Work out the finished part from the listing and answer in its coordinate system (mm). Give positions to 0.01 mm unless a question says otherwise; leave off trailing zeros. Loops run counter-clockwise (first coordinate to the right, second up) from the corner with the lowest first, then second, coordinate; pieces in that order, holes last. Notation, with made-up numbers: M -29,81.5 L -7,81.5 A23 cw -7,113.5 Z; hole C 45.5,0 d6. An arc over 180 degrees is marked long. Answer as a JSON object with one key per item and string values. Group by question number.
```python
from build123d import *

# Parameters (mm, degrees)
SKETCH1_W           = 25
SKETCH1_H           = 95
BOSS_EXTRUDE1_DEPTH = 1
BOSS_EXTRUDE2_START = -0.5
SKETCH3_W           = 3
SKETCH3_H           = 1
SKETCH3_W_2         = 1
SKETCH3_H_2         = 3
BOSS_EXTRUDE2_DEPTH = 0.5
SKETCH4_R           = 5
CUT_EXTRUDE1_DEPTH  = 1


with BuildPart() as part:
    # Sketch1 → Boss-Extrude1 (new body)
    with BuildSketch(Plane.XZ.offset(-34.2740501)):
        with Locations((-81.601257217, 49.307503177)):
            Rectangle(SKETCH1_W, SKETCH1_H)
    extrude(amount=-BOSS_EXTRUDE1_DEPTH)

    # Sketch3 → Boss-Extrude2 (add)
    with BuildSketch(Plane.XZ.offset(-34.2740501).offset(BOSS_EXTRUDE2_START)):
        with Locations((-81.601257217, 96.807503177)):
            Rectangle(SKETCH3_W, SKETCH3_H)
        with Locations((-94.101257217, 68.580262086)):
            Rectangle(SKETCH3_W_2, SKETCH3_H_2)
        with Locations((-94.101257217, 43.580262086)):
            Rectangle(SKETCH3_W_2, SKETCH3_H_2)
        with Locations((-94.101257217, 18.580262086)):
            Rectangle(SKETCH3_W_2, SKETCH3_H_2)
        with Locations((-69.101257217, 18.580262086)):
            Rectangle(SKETCH3_W_2, SKETCH3_H_2)
        with Locations((-69.101257217, 43.580262086)):
            Rectangle(SKETCH3_W_2, SKETCH3_H_2)
        with Locations((-69.101257217, 68.580262086)):
            Rectangle(SKETCH3_W_2, SKETCH3_H_2)
    extrude(amount=-BOSS_EXTRUDE2_DEPTH)

    # Sketch4 → Cut-Extrude1 (cut)
    with BuildSketch(Plane.XZ.offset(-34.2740501)):
        with Locations((-81.601257217, 1.807503177)):
            Circle(SKETCH4_R)
    extrude(amount=-CUT_EXTRUDE1_DEPTH, mode=Mode.SUBTRACT)


solid = part.part
```
Item 1: For a pull along X with two mould halves and no side action, classify faces 1 (the cylindrical face through (-81.491, 34.767, 6.806)), 2 (the flat face through (-82, 35.274, 50)) as pulls with the +X half, pulls with the -X half, needs draft (parallel to the pull), parting line crosses it, or undercut.
Item 2: Find the intervals of material crossed by probe 1 along Z at (x, y) = (-74.75, 35.2); probe 2 along X at (y, z) = (34.9, 38.5); probe 3 along X at (y, z) = (34.65, 6), in increasing order. Write a range as [from, to].
Item 3: Given pin 1 Ø0.6 at (x, y) = (-94.5, 35) entering from -Z; pin 2 Ø0.5 at (x, y) = (-76, 34.5) entering from +Z, each flat-ended and moving along its own axis, determine where each tip first touches the part or whether it passes through.
Item 4: A cutting plane is placed at C-C (x = -81.5). Determine the outline of the cut face in (y, z), and give its area (3 significant figures).
Item 5: A cutting plane is placed at D-D (x = -85.75). Determine the outline of the cut face in (y, z), and give its area (3 significant figures).
Item 6: A cutting plane is placed at B-B (z = 64.5). Determine the outline of the cut face in (x, y), and give its area (3 significant figures).
The answers:
{
 "1": {"face 1": "undercut", "face 2": "needs draft"},
 "2": {"probe 1": "z = [1.81, 96.81]", "probe 2": "x = [-94.1, -69.1]", "probe 3": "x = [-94.1, -84.33], [-78.88, -69.1]"},
 "3": {"pin 1": "stops at z = 17.08", "pin 2": "stops at z = 96.81"},
 "4": {"outline": "M 34.27,6.81 L 35.27,6.81 L 35.27,97.31 L 34.77,97.31 L 34.77,96.81 L 34.27,96.81 Z", "area": "90.3 mm^2"},
 "5": {"outline": "M 34.27,4.6 L 35.27,4.6 L 35.27,96.81 L 34.27,96.81 Z", "area": "92.2 mm^2"},
 "6": {"outline": "M -94.1,34.27 L -69.1,34.27 L -69.1,35.27 L -94.1,35.27 Z", "area": "25.0 mm^2"}
}
